Here's how the part is built. I have some questions about the finished solid (model axes, mm). A direction names the side the tool comes from. Coordinates: 2 decimals unless noted, no trailing zeros. Write each loop counter-clockwise with the first axis right and the second up, starting at its lowest first coordinate (ties: lowest second). Pieces come first, ordered by that corner, then holes. Notation, with made-up numbers: (79, 72.5) -> (96, 72.5) arc R26 ccw to (96, 90.5) -> close; hole circle Ø5 at (-24.5, 82). An arc over 180 degrees is marked (long way). Put each result on its own line as item: value.
```python
from build123d import *

# Parameters (mm, degrees)
F0_W     = 20
F0_H     = 20
F1_DEPTH = 4
F2_DEPTH = 5
F3_DEPTH = 5


with BuildPart() as f1:
    # F0 (on Top) → F1 (new body)
    with BuildSketch(Plane.XY):
        with Locations((-40.693533, -4.456982)):
            Rectangle(F0_W, F0_H)
        with BuildLine():
            Line((-48.125807, -4.26834), (-48.125807, 2.291039))
            Line((-48.125807, 2.291039), (-40.693533, 4.543018))
            Line((-40.693533, 4.543018), (-33.261258, 2.291039))
            Line((-33.261258, 2.291039), (-33.261258, -4.26834))
            add(Edge.make_bspline(
                [(-33.261258, -4.26834), (-34.245458, -8.461894), (-36.694674, -11.414499), (-40.693533, -13.456982)],
                knots=[0, 0, 0, 0, 11.8182, 11.8182, 11.8182, 11.8182], degree=3))
            add(Edge.make_bspline(
                [(-48.125807, -4.26834), (-47.141608, -8.461894), (-44.692392, -11.414499), (-40.693533, -13.456982)],
                knots=[0, 0, 0, 0, 11.8182, 11.8182, 11.8182, 11.8182], degree=3))
        make_face(mode=Mode.SUBTRACT)
    extrude(amount=F1_DEPTH)

    # F0 (on Top) → F2 (join)
    with BuildSketch(Plane.XY):
        with BuildLine():
            Line((-40.693533, 4.543018), (-48.125807, 2.291039))
            Line((-48.125807, 2.291039), (-48.125807, -4.26834))
            add(Edge.make_bspline(
                [(-48.125807, -4.26834), (-47.141608, -8.461894), (-44.692392, -11.414499), (-40.693533, -13.456982)],
                knots=[0, 0, 0, 0, 11.8182, 11.8182, 11.8182, 11.8182], degree=3))
            add(Edge.make_bspline(
                [(-33.261258, -4.26834), (-34.245458, -8.461894), (-36.694674, -11.414499), (-40.693533, -13.456982)],
                knots=[0, 0, 0, 0, 11.8182, 11.8182, 11.8182, 11.8182], degree=3))
            Line((-33.261258, -4.26834), (-33.261258, 2.291039))
            Line((-33.261258, 2.291039), (-40.693533, 4.543018))
        make_face()
        with BuildLine():
            Line((-40.693533, 3.262941), (-40.693533, -12.135648))
            add(Edge.make_bspline(
                [(-40.693533, -12.135648), (-44.436548, -10.041109), (-47.01202, -6.495423), (-47.08004, -3.659984)],
                knots=[0, 0, 0, 0, 10.612463, 10.612463, 10.612463, 10.612463], degree=3))
            Line((-47.08004, -3.659984), (-47.08004, 1.440438))
            Line((-47.08004, 1.440438), (-40.693533, 3.340149))
            Line((-40.693533, 3.340149), (-40.693533, 3.262941))
        make_face(mode=Mode.SUBTRACT)
    extrude(amount=F2_DEPTH)

    # F0 (on Top) → F3 (join)
    with BuildSketch(Plane.XY):
        with BuildLine():
            add(Edge.make_bspline(
                [(-40.693533, -12.135648), (-44.436548, -10.041109), (-47.01202, -6.495423), (-47.08004, -3.659984)],
                knots=[0, 0, 0, 0, 10.612463, 10.612463, 10.612463, 10.612463], degree=3))
            Line((-40.693533, -12.135648), (-40.693533, 3.262941))
            Line((-40.693533, 3.262941), (-40.693533, 3.340149))
            Line((-40.693533, 3.340149), (-47.08004, 1.440438))
            Line((-47.08004, 1.440438), (-47.08004, -3.659984))
        make_face()
    extrude(amount=F3_DEPTH)


solid = f1.part
```
Item 1: Imagine slicing it at A-A on y = -3.5. Write out the boundary of the cut face in (x, z), then the cut area to 3 significant figures.
Output:
outline: (-50.69, 0) -> (-30.69, 0) -> (-30.69, 4) -> (-33.26, 4) -> (-33.26, 5) -> (-48.13, 5) -> (-48.13, 4) -> (-50.69, 4) -> close
area: 94.9 mm²
Item 2: Imagine slicing it at B-B on x = -48.5. Write out the boundary of the cut face in (y, z), then the cut area to 3 significant figures.
Output:
outline: (-14.46, 0) -> (5.54, 0) -> (5.54, 4) -> (-14.46, 4) -> close
area: 80.0 mm²
Item 3: Please list where these lines run through material, in increasing order: line 1 along Z through (x, y) = (-31.75, -4); line 2 along X through (y, z) = (-12.75, 4.7). Write a range as from..to.
Output:
line 1: z = 0..4
line 2: x = -41.96..-39.43
Item 4: For P1, Ø0.8, axis at y = -2, z = 4.5, coming from the +X side; P2, Ø0.8, axis at y = -0.5, z = 4.5, coming from the -X side, each with a flat end and sliding along its axis, tell me the tip position at first contact or that it passes through.
Output:
P1: stops at x = -33.26
P2: stops at x = -48.13
Item 5: Imagine slicing it at C-C on y = 3.25. Write out the boundary of the cut face in (x, z).
Output:
outline: (-50.69, 0) -> (-30.69, 0) -> (-30.69, 4) -> (-36.43, 4) -> (-36.43, 5) -> (-44.96, 5) -> (-44.96, 4) -> (-50.69, 4) -> close
Item 6: Which directions (+Z, -Z, +X, -X, +Y, -Y) give clear straight access to the entire face, cutting with the end or side of a thin tool? Please do faces 1 (the flat face through (-48.126, -0.9, 4.5)), 2 (the flat face through (-33.261, -1, 4.5)), 3 (the flat face through (-48, -7, 4)), 4 (the flat face through (-44.36, 3.43, 4.49)).
Output:
face 1: +Z, -X, +Y, -Y
face 2: +Z, +X, +Y, -Y
face 3: +Z
face 4: +Z, -X, +Y
